Job drawing, mm, ordinate dimensions from the low corner. One solid piece. A direction names the side the tool comes from. Round coordinates to 2 decimals unless told otherwise and drop trailing zeros. Write each loop counter-clockwise with the first axis right and the second up, starting at its lowest first coordinate (ties: lowest second). Pieces come first, ordered by that corner, then holes. Notation, with made-up numbers: (26.5, 14.25) -> (49.5, 14.25) arc R18 cw to (49.5, 29.25) -> close; hole circle Ø5 at (22.5, 44.25). An arc over 180 degrees is marked (long way). Use CSV: the item, a comma, the result in double quotes. Start each with the question number.
(1) Saw through at D-D (x = 47). Give the cut face in (y, z).
(2) Probe line 1 (X direction, y = 11, z = 10); line 2 (X direction, y = 13.5, z = 4.75); line 3 (Z direction, x = 58, y = 8.5). List the from-to ranges inside material, lowest first. Write a range as [from, to].
(3) Saw through at B-B (x = 62.5). Give the cut face in (y, z), plus the area to 3 significant figures.
(4) Saw through at C-C (z = 8.75). Give the cut face in (x, y), plus the area to 3 significant figures.
(5) Saw through at A-A (z = 5.25). Give the cut face in (x, y).
(6) Which spindle directions (+Z, -Z, +X, -X, +Y, -Y) get a long thin tool onto all of the face, cutting with end or side? Do the marked faces 4, 5, 6, 7 and 8. Say none if no direction does.
(7) Two-plate mould, pull along Z, no slides. Class the marked faces 1, 2 and 3: released by +Z, released by -Z, zero draft, split by the parting line, or undercut.
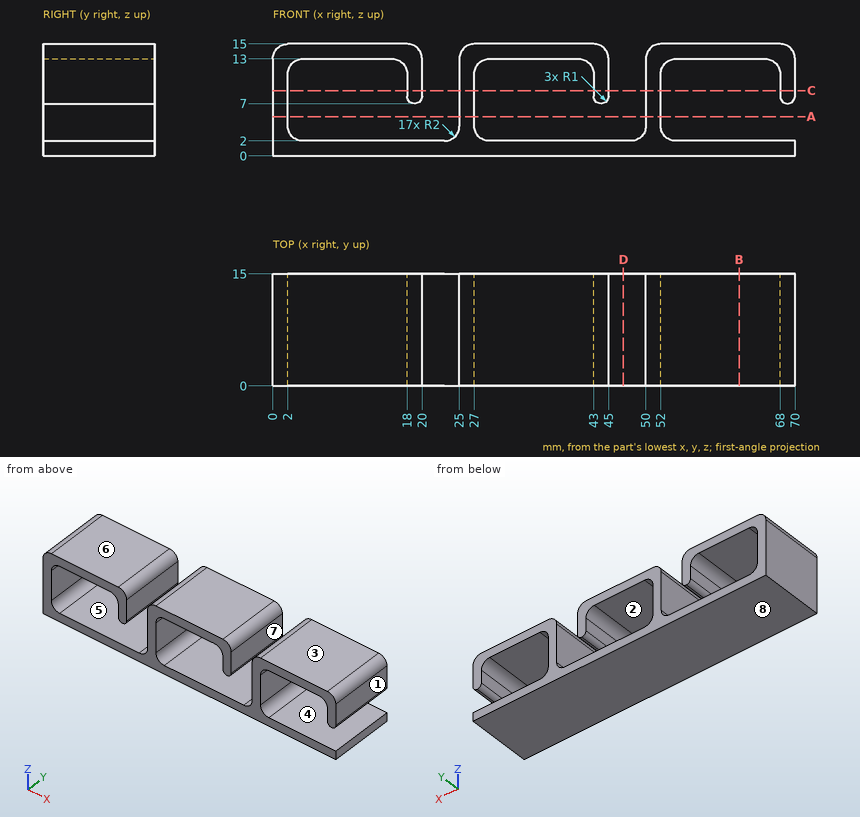
Answers:
1,outline,"(0, 0) -> (15, 0) -> (15, 2) -> (0, 2) -> close"
2,line 1,"x = [0, 2], [18, 20], [25, 27], [43, 45], [50, 52], [68, 70]"
2,line 2,"x = [0, 2], [25, 27], [50, 52]"
2,line 3,"z = [0, 2], [13, 15]"
3,outline,"(0, 0) -> (15, 0) -> (15, 2) -> (0, 2) -> close; (0, 13) -> (15, 13) -> (15, 15) -> (0, 15) -> close"
3,area,"60.0 mm²"
4,outline,"(0, 0) -> (2, 0) -> (2, 15) -> (0, 15) -> close; (18, 0) -> (20, 0) -> (20, 15) -> (18, 15) -> close; (25, 0) -> (27, 0) -> (27, 15) -> (25, 15) -> close; (43, 0) -> (45, 0) -> (45, 15) -> (43, 15) -> close; (50, 0) -> (52, 0) -> (52, 15) -> (50, 15) -> close; (68, 0) -> (70, 0) -> (70, 15) -> (68, 15) -> close"
4,area,"180 mm²"
5,outline,"(0, 0) -> (2, 0) -> (2, 15) -> (0, 15) -> close; (25, 0) -> (27, 0) -> (27, 15) -> (25, 15) -> close; (50, 0) -> (52, 0) -> (52, 15) -> (50, 15) -> close"
6,face 4,"+X, +Y, -Y"
6,face 5,"+Y, -Y"
6,face 6,"+Z, +X, -X, +Y, -Y"
6,face 7,"+Z, +Y, -Y"
6,face 8,"-Z, +X, -X, +Y, -Y"
7,face 1,"zero draft"
7,face 2,"undercut"
7,face 3,"released by +Z"
